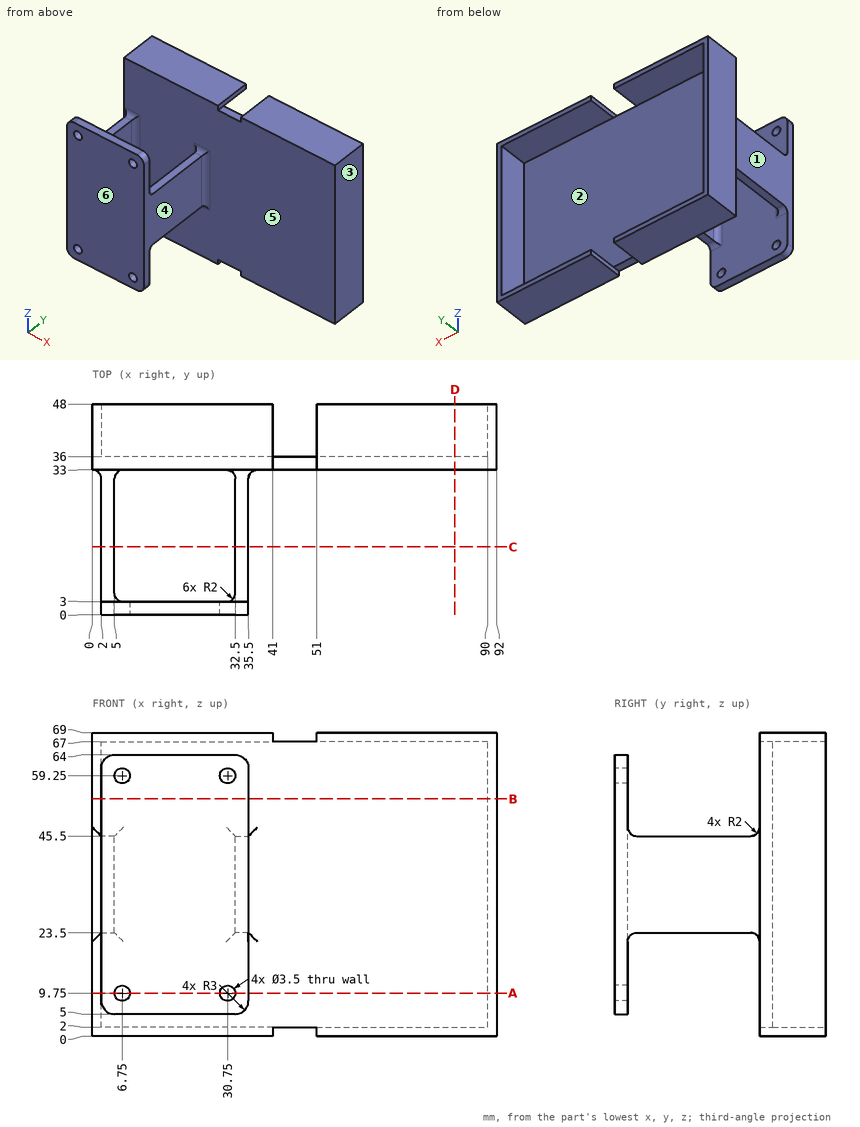
Geometry: see drawing. Coordinates: mm, zero at the bounding-box minimum. A direction names the side the tool comes from. Round coordinates to 2 decimals unless told otherwise and drop trailing zeros. Write each loop counter-clockwise with the first axis right and the second up, starting at its lowest first coordinate (ties: lowest second). Pieces come first, ordered by that corner, then holes. Notation, with made-up numbers: M 47.25,20 L 90.25,20 A26 ccw 90.25,36 Z; hole C 87.25,54 d5. An arc over 180 degrees is marked long. Answer as a JSON object with one key per item and string values. Group by question number.
(1) Section query C-C on y = 15.5. Output: boundary loops of the cut face in (x, z), then the cut area to 3 significant figures.
(2) Reachability of the marked faces 1, 2 and 3 from +Z, -Z, +X, -X, +Y, -Y: full face, straight path, thin tool, end or side. Return the list, or none.
(3) First-contact query: pin 1 (3 mm diameter, centred on x = 6.75, z = 9.75, fed in from -Y); pin 2 (0.9 mm diameter, centred on x = 33.5, y = 16.5, fed in from +Z); pin 3 (4 mm diameter, centred on x = 67, z = 25, fed in from +Y). Flat tips, straight axial feed; report the tip coordinate or a pass-through.
(4) Ray query, line 1 (Z direction, x = 30.75, y = 0.6); line 2 (X direction, y = 43, z = 14); line 3 (Z direction, x = 75, y = 40). Return the intervals inside material, ascending. Write a range as [from, to].
(5) Section query A-A on z = 9.75. Output: boundary loops of the cut face in (x, y).
(6) Section query D-D on x = 82.5. Output: boundary loops of the cut face in (y, z).
(7) Section query B-B on z = 54. Output: boundary loops of the cut face in (x, y).
(8) Mould query, pull axis Y, two halves, no side actions, for the marked faces 4, 5 and 6. Classes: +Y half, -Y half, draft (parallel to the pull), parting line (faces both ways), or undercut.
Computed values:
{
 "1": {"outline": "M 2,23.5 L 5,23.5 L 5,45.5 L 2,45.5 Z; M 32.5,23.5 L 35.5,23.5 L 35.5,45.5 L 32.5,45.5 Z", "area": "132 mm^2"},
 "2": {"face 1": "+Z, -Z, -X, -Y", "face 2": "+Y", "face 3": "+Z, -Z, +X, +Y, -Y"},
 "3": {"pin 1": "y = 33", "pin 2": "z = 45.5", "pin 3": "y = 36"},
 "4": {"line 1": "[5, 8], [11.5, 57.5], [61, 64]", "line 2": "[0, 2], [90, 92]", "line 3": "[0, 2], [67, 69]"},
 "5": {"outline": "M 0,33 L 92,33 L 92,48 L 90,48 L 90,36 L 2,36 L 2,48 L 0,48 Z; M 2,0 L 5,0 L 5,3 L 2,3 Z; M 8.5,0 L 29,0 L 29,3 L 8.5,3 Z; M 32.5,0 L 35.5,0 L 35.5,3 L 32.5,3 Z"},
 "6": {"outline": "M 33,0 L 48,0 L 48,2 L 36,2 L 36,67 L 48,67 L 48,69 L 33,69 Z"},
 "7": {"outline": "M 0,33 L 92,33 L 92,48 L 90,48 L 90,36 L 2,36 L 2,48 L 0,48 Z; M 2,0 L 35.5,0 L 35.5,3 L 2,3 Z"},
 "8": {"face 4": "draft", "face 5": "undercut", "face 6": "-Y half"}
}
